CAD build for the part. Positions are in the model's coordinates, mm. Face numbers are marked on the shaded views. A direction names the side the tool comes from. Round coordinates to 2 decimals unless told otherwise and drop trailing zeros. Write each loop counter-clockwise with the first axis right and the second up, starting at its lowest first coordinate (ties: lowest second). Pieces come first, ordered by that corner, then holes. Notation, with made-up numbers: (81, 61) - (135, 61) arc R26 ccw to (135, 76) - close; hole circle Ø7 at (43.5, 61). An arc over 180 degrees is marked (long way). Use one line per item in the form item = value. Start each with the question number.
Item 1: Drill centre lines: L1, parallel to Y at x = -68, z = 3.4; L2, parallel to Y at x = -30, z = 5.2; L3, parallel to Y at x = -69, z = 1.45. Where is each one in solid material? Low to high.
Item 2: Band-saw the part on C-C, the plane x = -32.5. List the corners of the cut face in (y, z), and give its area (3 significant figures).
Item 3: Tool access for the marked faces 1 and 2: list every direction of +Z, -Z, +X, -X, +Y, -Y with a clear straight run to the whole face (end or side of a thin tool).
Item 4: Band-saw the part on D-D, the plane y = 3.5. List the corners of the cut face in (x, z).
Item 5: Pin check, flat tips, straight feed: pin 1 (4 mm diameter, centred on x = -30.33, y = -41.75, fed in from +Z); pin 2 (2 mm diameter, centred on y = 28.5, z = 2, fed in from +X); pin 3 (3 mm diameter, centred on x = -69, z = 2, fed in from +Y). Stop position of each tip, or through.
Item 6: Band-saw the part on B-B, the plane z = 1.55. List the corners of the cut face in (x, y), and give its area (3 significant figures).
Item 7: Pull direction Y, two halves, no side cores. Call the marked faces 3, 4, 5 and 6: +Y half, -Y half, draft (parallel to the pull), parting line (faces both ways), or undercut.
Item 8: Band-saw the part on A-A, the plane x = -68. List the corners of the cut face in (y, z).
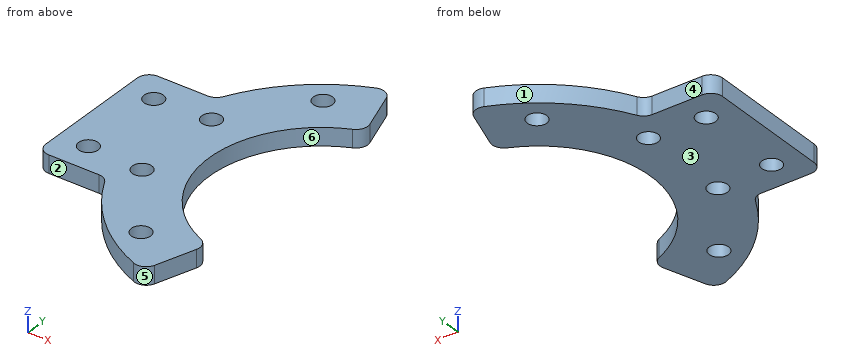
from build123d import *

# Parameters (mm, degrees)
SKETCH1_R           = 3.3
BOSS_EXTRUDE1_DEPTH = 6


with BuildPart() as part:
    # Sketch1 → Boss-Extrude1 (new body)
    with BuildSketch(Plane.XY):
        with BuildLine():
            Line((-17.260749948, 53.123125955), (-12.919719305, 39.762807409))
            ThreePointArc((-12.919719305, 39.762807409), (-13.077398812, 36.882750928), (-15.131188668, 34.857526153))
            ThreePointArc((-15.131188668, 34.857526153), (-38, 0), (-15.131188668, -34.857526153))
            ThreePointArc((-15.131188668, -34.857526153), (-13.077398812, -36.882750928), (-12.919719305, -39.762807409))
            Line((-12.919719305, -39.762807409), (-17.260749948, -53.123125955))
            ThreePointArc((-17.260749948, -53.123125955), (-19.377542011, -55.513704705), (-22.569617157, -55.593276404))
            ThreePointArc((-22.569617157, -55.593276404), (-40.59393325, -44.182944485), (-53.486819346, -27.1875))
            ThreePointArc((-53.486819346, -27.1875), (-54.960957236, -25.590454576), (-57.052607302, -25))
            Line((-57.052607302, -25), (-74, -25))
            ThreePointArc((-74, -25), (-76.828427125, -23.828427125), (-78, -21))
            Line((-78, -21), (-78, 21))
            ThreePointArc((-78, 21), (-76.828427125, 23.828427125), (-74, 25))
            Line((-74, 25), (-57.052607302, 25))
            ThreePointArc((-57.052607302, 25), (-54.960957236, 25.590454576), (-53.486819346, 27.1875))
            ThreePointArc((-53.486819346, 27.1875), (-40.59393325, 44.182944485), (-22.569617157, 55.593276404))
            ThreePointArc((-22.569617157, 55.593276404), (-19.377542011, 55.513704705), (-17.260749948, 53.123125955))
        make_face()
        with Locations((-30.329719018, -41.74527691)):
            Circle(SKETCH1_R, mode=Mode.SUBTRACT)
        with Locations((-49.074516241, -15.94527691)):
            Circle(SKETCH1_R, mode=Mode.SUBTRACT)
        with Locations((-49.074516241, 15.94527691)):
            Circle(SKETCH1_R, mode=Mode.SUBTRACT)
        with Locations((-30.329719018, 41.74527691)):
            Circle(SKETCH1_R, mode=Mode.SUBTRACT)
        with Locations((-68, 15)):
            Circle(SKETCH1_R, mode=Mode.SUBTRACT)
        with Locations((-68, -15)):
            Circle(SKETCH1_R, mode=Mode.SUBTRACT)
    extrude(amount=BOSS_EXTRUDE1_DEPTH)


solid = part.part
Determined:
q1.L1 = -25 to -18.3, -11.7 to 11.7, 18.3 to 25
q1.L2 = -51.96 to -45.03, -38.46 to -23.32, 23.32 to 38.46, 45.03 to 51.96
q1.L3 = -25 to -18.14, -11.86 to 11.86, 18.14 to 25
q2.outline = (-50.44, 0) - (-44.23, 0) - (-44.23, 6) - (-50.44, 6) - close; (-39.26, 0) - (-19.69, 0) - (-19.69, 6) - (-39.26, 6) - close; (19.69, 0) - (39.26, 0) - (39.26, 6) - (19.69, 6) - close; (44.23, 0) - (50.44, 0) - (50.44, 6) - (44.23, 6) - close
q2.area = 309 mm²
q3.face_1 = +Z, -Z, -X, +Y
q3.face_2 = +Z, -Z, -X, -Y
q4.outline = (-78, 0) - (-37.84, 0) - (-37.84, 6) - (-78, 6) - close
q5.pin_1 = through
q5.pin_2 = -23.95
q5.pin_3 = 25
q6.outline = (-78, -21) arc R4 ccw to (-74, -25) - (-57.05, -25) arc R4 cw to (-53.49, -27.19) arc R60 ccw to (-22.57, -55.59) arc R4 ccw to (-17.26, -53.12) - (-12.92, -39.76) arc R4 ccw to (-15.13, -34.86) arc R38 cw to (-15.13, 34.86) arc R4 ccw to (-12.92, 39.76) - (-17.26, 53.12) arc R4 ccw to (-22.57, 55.59) arc R60 ccw to (-53.49, 27.19) arc R4 cw to (-57.05, 25) - (-74, 25) arc R4 ccw to (-78, 21) - close; hole circle Ø6.6 at (-68, -15); hole circle Ø6.6 at (-68, 15); hole circle Ø6.6 at (-49.07, -15.95); hole circle Ø6.6 at (-49.07, 15.95); hole circle Ø6.6 at (-30.33, -41.75); hole circle Ø6.6 at (-30.33, 41.75)
q6.area = 3,470 mm²
q7.face_3 = draft
q7.face_4 = +Y half
q7.face_5 = -Y half
q7.face_6 = undercut
q8.outline = (-25, 0) - (-18.3, 0) - (-18.3, 6) - (-25, 6) - close; (-11.7, 0) - (11.7, 0) - (11.7, 6) - (-11.7, 6) - close; (18.3, 0) - (25, 0) - (25, 6) - (18.3, 6) - close
